Check sheet for the modelled part. Datum: model origin and axes. Units: mm. Face numbers are marked on the shaded views. A direction names the side the tool comes from. Round coordinates to 2 decimals unless told otherwise and drop trailing zeros. Order: outer loops, then holes, each group sorted by start corner. A loop starts at its lowest first (then second) coordinate and runs counter-clockwise, first axis right, second up. Notation, with made-up numbers: (18, 5.25) -> (55, 5.25) arc R26 cw to (55, 31.25) -> close; hole circle Ø4 at (52, -20.75). An arc over 180 degrees is marked (long way). Answer in a Markdown table with one row per item. Add a question column.
1. Access from +Z, -Z, +X, -X, +Y, -Y to the whole of each face (thin tool, end or side, straight path). Record for the marked faces 1, 2, 3 and 4.
2. Sectioned sample at D-D, the plane y = -7. Record the boundary of the cut face in (x, z), then the cut area to 3 significant figures.
3. Sectioned sample at C-C, the plane z = -380. Record the boundary of the cut face in (x, y), then the cut area to 3 significant figures.
4. Sectioned sample at B-B, the plane z = -29.5. Record the boundary of the cut face in (x, y), then the cut area to 3 significant figures.
5. Depth check by flat-ended pin: P1, Ø4, axis at x = -10.5, y = -2, coming from the +Z side; P2, Ø22.5, axis at x = -3, z = -149.5, coming from the +Y side; P3, Ø22.5, axis at x = 9.5, z = -37, coming from the -Y side. Enter the tip coordinate at first touch or a pass-through.
6. Sectioned sample at A-A, the plane x = 17.5. Record the boundary of the cut face in (y, z), then the cut area to 3 significant figures.
7. Material ranges on L1, parallel to Z at x = 0, y = 14.5; L2, parallel to Z at x = 0, y = -17.75; L3, parallel to X at y = -14, z = 0, recorded low to high. Write a range as from..to.
Autodesk Inventor part; units mm, degrees
ref_plane "YZ Plane" through (0, 0, 0) normal (1, 0, 0) x (0, 1, 0)
ref_plane "XZ Plane" through (0, 0, 0) normal (0, 1, 0) x (-1, 0, 0)
ref_plane "XY Plane" through (0, 0, 0) normal (0, 0, 1) x (1, 0, 0)
sketch "Sketch1" plane through (0, 0, 0) normal (1, 0, 0) x (0, 1, 0)
  circle A0 centre (0, 0) radius 10
  circle A1 centre (-380, 0) radius 10
  line L0 (0, 0) -> (-380, 0) construction
  line L1 (20, 22.5) -> (-400, 22.5)
  line L2 (-400, 22.5) -> (-400, -22.5)
  line L3 (-400, -22.5) -> (20, -22.5)
  line L4 (20, -22.5) -> (20, 22.5)
  line L5 (20, 0) -> (-400, 0) construction
  dimension "d0" = 380
  dimension "d2" = 20
  dimension "d3" = 20
  dimension "d4" = 20
  dimension "d5" = 20
  dimension "d6" = 45
extrude "Extrusion1" add sketch "Sketch1" along normal mid plane 24
sketch "Sketch2" plane through (12, 0, 0) normal (1, 0, 0) x (0, 0, -1)
  circle A0 centre (0, 0) radius 10
  line L0 (22.5, -400) -> (22.5, 20)
  line L1 (22.5, 20) -> (-22.5, 20)
  line L2 (-22.5, 20) -> (22.5, 20)
  line L3 (22.5, 20) -> (22.5, -90)
  line L4 (22.5, -90) -> (-22.5, -90)
  line L5 (-22.5, -90) -> (-22.5, 20)
  circle A1 centre (0, 0) radius 10
  dimension "d9" = 110
extrude "Extrusion2" add sketch "Sketch2" along normal blind 10
mirror "Mirror1" about plane through (0, 0, 0) normal (1, 0, 0) of "Extrusion2"
sketch "Sketch3" plane through (-12, -400, 22.5) normal (0, 0, 1) x (1, 0, 0)
  line L0 (34, 420) -> (-10, 420)
  line L1 (0, 420) -> (24, 420)
  line L2 (24, 420) -> (24, 345)
  line L3 (24, 345) -> (0, 345)
  line L4 (0, 345) -> (0, 420)
  line L5 (12, 420) -> (12, 345) construction
  point P0 (12, 400)
  dimension "d12" = 24
  dimension "d14" = 75
extrude "Extrusion3" cut sketch "Sketch3" against normal through all
sketch "Sketch4" plane through (12, 0, 0) normal (1, 0, 0) x (0, 0, -1)
  line L0 (22.5, -400) -> (22.5, -90)
  circle A0 centre (0, -380) radius 10
  line L1 (-22.5, -400) -> (22.5, -400)
  line L2 (22.5, -400) -> (22.5, -295)
  line L3 (22.5, -295) -> (-22.5, -295)
  line L4 (-22.5, -295) -> (-22.5, -400)
  circle A1 centre (0, -380) radius 10
  point P0 (0, 0)
  dimension "d18" = 85
extrude "Extrusion4" add sketch "Sketch4" along normal blind 15.5
mirror "Mirror2" about plane through (0, 0, 0) normal (1, 0, 0) of "Extrusion4"
sketch "Sketch5" plane through (22, -90, 22.5) normal (0, 0, 1) x (1, 0, 0)
  line L0 (-49.5, -310) -> (5.5, -310)
  line L1 (-39.5, -310) -> (-4.5, -310)
  line L2 (-4.5, -310) -> (-4.5, -252)
  line L3 (-4.5, -252) -> (-39.5, -252)
  line L4 (-39.5, -252) -> (-39.5, -310)
  line L5 (-22, -252) -> (-22, -310) construction
  point P0 (-22, 90)
  point P1 (-22, -310)
  dimension "d21" = 35
  dimension "d23" = 58
extrude "Extrusion5" cut sketch "Sketch5" against normal through all
move or copy body "Move Body1" bodies to move or copy 1 copy no rotation origin (0, 0, 0) rotation axis (1, 0, 0) rotation angle 90
move or copy body "Move Body2" bodies to move or copy 1 copy no rotation origin (0, 0, 0) rotation axis (0, 0, 1) rotation angle 90
properties part number "LowerLeg_v2"
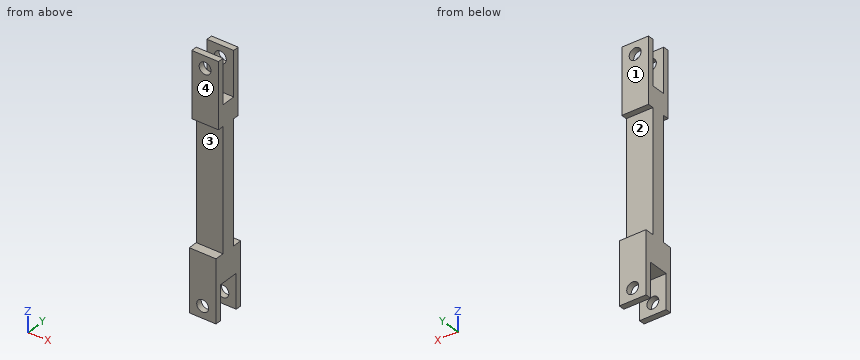
Answer key:
| question | item | result |
|---|---|---|
| 1 | face 1 | +Z, +X, -X, +Y |
| 1 | face 2 | +X, -X, +Y |
| 1 | face 3 | +X, -X, -Y |
| 1 | face 4 | +Z, +X, -X, -Y |
| 2 | outline | (-22.5, -342) -> (22.5, -342) -> (22.5, -55) -> (-22.5, -55) -> close |
| 2 | area | 12,900 mm² |
| 3 | outline | (-22.5, -27.5) -> (-10, -27.5) -> (-10, -17.5) -> (-22.5, -17.5) -> close; (-22.5, 17.5) -> (-10, 17.5) -> (-10, 27.5) -> (-22.5, 27.5) -> close; (10, -27.5) -> (22.5, -27.5) -> (22.5, -17.5) -> (10, -17.5) -> close; (10, 17.5) -> (22.5, 17.5) -> (22.5, 27.5) -> (10, 27.5) -> close |
| 3 | area | 500 mm² |
| 4 | outline | (-22.5, -22) -> (22.5, -22) -> (22.5, -12) -> (-22.5, -12) -> close; (-22.5, 12) -> (22.5, 12) -> (22.5, 22) -> (-22.5, 22) -> close |
| 4 | area | 900 mm² |
| 5 | P1 | stops at z = -55 |
| 5 | P2 | stops at y = 12 |
| 5 | P3 | stops at y = -22 |
| 6 | outline | (-27.5, -400) -> (-17.5, -400) -> (-17.5, -342) -> (17.5, -342) -> (17.5, -400) -> (27.5, -400) -> (27.5, -295) -> (12, -295) -> (12, -90) -> (22, -90) -> (22, 20) -> (12, 20) -> (12, -55) -> (-12, -55) -> (-12, 20) -> (-22, 20) -> (-22, -90) -> (-12, -90) -> (-12, -295) -> (-27.5, -295) -> close |
| 6 | area | 11,700 mm² |
| 7 | L1 | z = -342..-295, -90..-10, 10..20 |
| 7 | L2 | z = -400..-390, -370..-295, -90..-10, 10..20 |
| 7 | L3 | x = -22.5..-10, 10..22.5 |
